CAD build for the part. Positions are in the model's coordinates, mm. Coordinates: 2 decimals unless noted, no trailing zeros. Order: outer loops, then holes, each group sorted by start corner. A loop starts at its lowest first (then second) coordinate and runs counter-clockwise, first axis right, second up. Notation, with made-up numbers: (60, 38.25) - (107, 38.25) arc R7 cw to (107, 43.25) - close; hole circle Ø3 at (57.5, 50). An arc over 180 degrees is marked (long way). Return JSON: item names as keys, results as strings.
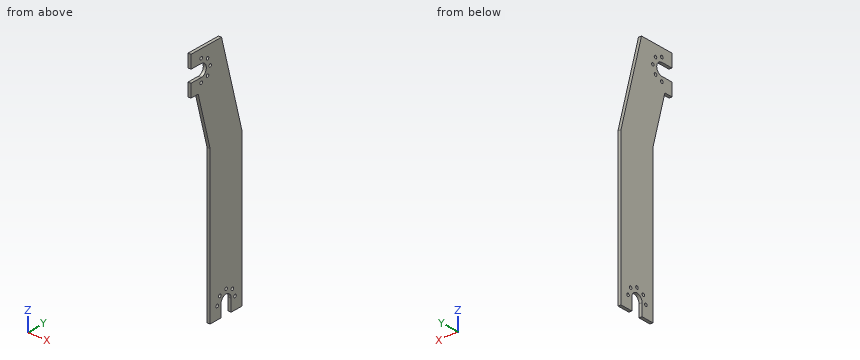
Autodesk Inventor part; units mm, degrees
ref_plane "YZ Plane" through (0, 0, 0) normal (1, 0, 0) x (0, 1, 0)
ref_plane "XZ Plane" through (0, 0, 0) normal (0, 1, 0) x (-1, 0, 0)
ref_plane "XY Plane" through (0, 0, 0) normal (0, 0, 1) x (1, 0, 0)
sketch "スケッチ1" plane through (0, 0, 0) normal (1, 0, 0) x (0, 1, 0)
  line L0 (-20, 80) -> (20, 80)
  line L1 (20, 80) -> (20, -80)
  line L2 (20, -80) -> (-20, -80)
  line L3 (-20, -80) -> (-20, 80)
  point P0 (0, 0)
  dimension "d0" = 40
  dimension "d2" = 160
  dimension "d3" = 80
  dimension "d4" = 20
extrude "押し出し1" add sketch "スケッチ1" along normal blind 2
sketch "スケッチ2" plane through (2, 0, 0) normal (1, 0, 0) x (0, 0, -1)
  line L0 (-80, 20) -> (-80, -20)
  line L1 (-80, -20) -> (80, -20)
  line L2 (80, -20) -> (80, 20)
  line L3 (80, 20) -> (-80, 20)
  line L4 (-80, 3.923) -> (-20, 20)
  line L5 (-55, -20) -> (-55, -14.3782)
  line L6 (-55, -14.3782) -> (-20, -5)
  line L7 (-20, -5) -> (80, -5)
  point P0 (0, 0)
  dimension "d7" = 25
  dimension "d8" = 165
  dimension "d9" = 15
  dimension "d10" = 100
  dimension "d11" = 100
  dimension "d12" = 25
extrude "押し出し2" cut sketch "スケッチ2" against normal blind 2 contours L4 L3 L2 L7 L6 L5 L1 L0 keep common part
sketch "スケッチ3" plane through (2, 0, 0) normal (1, 0, 0) x (0, 0, -1)
  line L0 (80, -5) -> (-20, -5)
  line L1 (80, -5) -> (80, 20)
  line L2 (80, 20) -> (-20, 20)
  line L3 (-80, 3.923) -> (-20, 20)
  line L4 (-80, 3.923) -> (-80, -20)
  line L5 (-80, -20) -> (-55, -20)
  line L6 (-55, -14.3782) -> (-55, -20)
  line L7 (-20, -5) -> (-55, -14.3782)
  line L8 (-71.5, -20) -> (-63.5, -20)
  line L9 (-63.5, -20) -> (-63.5, -12)
  line L10 (-71.5, -12) -> (-71.5, -20)
  line L11 (80, 11.5) -> (72, 11.5)
  line L12 (72, 3.5) -> (80, 3.5)
  line L13 (80, 3.5) -> (80, 11.5)
  arc A0 (-63.5, -12) -> (-71.5, -12) centre (-67.5, -12) ccw
  arc A1 (72, 11.5) -> (72, 3.5) centre (72, 7.5) ccw
  point P0 (0, 0)
  dimension "d18" = 8
  dimension "d19" = 12.5
  dimension "d20" = 8
  dimension "d21" = 12.5
  dimension "d23" = 8
  dimension "d24" = 4
  dimension "d25" = 8
  dimension "d26" = 8
  dimension "d27" = 8
extrude "押し出し3" cut sketch "スケッチ3" against normal blind 2 contours L0 L7 L6 L5 L9 A0 L10 L4 L3 L2 L1 L11 A1 L12 keep common part
sketch "スケッチ4" plane through (2, 0, 0) normal (1, 0, 0) x (0, 0, -1)
  arc A0 (72, 11.5) -> (72, 3.5) centre (72, 7.5) ccw
  line L0 (80, 11.5) -> (80, 20)
  line L1 (-80, -20) -> (-71.5, -20)
  arc A1 (-63.5, -12) -> (-71.5, -12) centre (-67.5, -12) ccw
  circle A2 centre (-74.5, -12) radius 1
  circle A3 centre (72, 14.5) radius 1
  point P0 (0, 0)
  dimension "d30" = 8
  dimension "d31" = 7
  dimension "d32" = 2
  dimension "d33" = 8
  dimension "d34" = 7
hole "穴1" at (2, -12, 74.5) at (2, 14.5, -72) direction (-1, 0, 0) diameter 2 end through all
pattern_circular "円形状パターン1" count 5 over 180 about axis through (2, -12, 67.5) along (-1, 0, 0) of "穴1"
pattern_circular "円形状パターン2" count 5 over 180 about axis through (2, 7.5, -72) along (1, 0, 0) of "穴1"
properties part number "Flame"
Item 1: Drop flat-ended pins along their axis: P1, Ø1.8, axis at y = 7.5, z = -65, coming from the -X side; P2, Ø1, axis at x = 1, z = -40, coming from the -Y side. Give the stop position or say it passes through.
Findings below:
{"P1": "passes through", "P2": "stops at y = -5"}
Item 2: Wall check: L1, parallel to Y at x = 1.6, z = -72; L2, parallel to Y at x = 1.3, z = 62; L3, parallel to Y at x = 0.85, z = 60.5. Give the ranges that are in metal, low to high. Write a range as [from, to].
Findings below:
{"L1": "y = [-5, -0.5], [1.5, 3.5], [11.5, 13.5], [15.5, 20]", "L2": "y = [-20, -7.89], [-6.22, 8.75]", "L3": "y = [-20, -13], [-11, 9.15]"}
Item 3: Band-saw the part on A-A, the plane z = 8. List the corners of the cut face in (x, y).
Findings below:
{"outline": "(0, -5) - (2, -5) - (2, 20) - (0, 20) - close"}
